Geometry check sheet. Reference: the model listing, model coordinates, mm. A direction names the side the tool comes from. Give positions to 0.01 mm unless a question says otherwise; leave off trailing zeros. Loops run counter-clockwise (first coordinate to the right, second up) from the corner with the lowest first, then second, coordinate; pieces in that order, holes last. Notation, with made-up numbers: (70.25, -39.75) -> (97.25, -39.75) arc R21 ccw to (97.25, -3.75) -> close; hole circle Ø3 at (50, 46.25). An arc over 180 degrees is marked (long way). Answer as a JSON object with one key per item and string values.
from build123d import *

# Parameters (mm, degrees)
BOSS_EXTRUDE1_DEPTH   = 3.175
F_6_CLEARANCE_HOLE1_D = 4.3053


with BuildPart() as part:
    # Sketch1 → Boss-Extrude1 (new body)
    with BuildSketch(Plane.XY):
        Polygon((866.156250481, 6490.011012461), (829.199261489, 6490.03953741), (829.199261489, 6625.537287847), (866.263292559, 6628.694971151), align=None)
        with BuildLine():
            Line((856.233206108, 6589.718701179), (856.176475752, 6516.218723072))
            ThreePointArc((856.176475752, 6516.218723072), (849.821576449, 6509.873626158), (843.476479535, 6516.22852546))
            Line((843.476479535, 6516.22852546), (843.533209891, 6589.728503567))
            ThreePointArc((843.533209891, 6589.728503567), (849.888109194, 6596.073600482), (856.233206108, 6589.718701179))
        make_face(mode=Mode.SUBTRACT)
    extrude(amount=BOSS_EXTRUDE1_DEPTH)

    # #6 Clearance Hole1 (through all)
    with Locations(Plane.XY.offset(3.175)):
        with Locations((859.90595224, 6619.187287847), (835.549261489, 6494.797137633)):
            Hole(F_6_CLEARANCE_HOLE1_D / 2)


solid = part.part
1) Draft check along X on faces 1 (the face through (840, 6560, 0)), 2 (the face through (829.199, 6557, 2)), 3 (the face through (835.83, 6496.93, 1.57)), 4 (the face through (858.91, 6617.28, 1.57)). Enter one of: pulls with the +X half, pulls with the -X half, needs draft (parallel to the pull), parting line crosses it, or undercut.
Geometry check:
{"face 1": "needs draft", "face 2": "pulls with the -X half", "face 3": "undercut", "face 4": "undercut"}
2) Tool access check on faces 5 (the face through (840, 6560, 3.175)), 6 (the face through (849.748, 6596.072, 1.565)). Record the directions out of +Z, -Z, +X, -X, +Y, -Y that give a thin tool (end or side, any length) a straight path to the whole face; none if there is none.
Geometry check:
{"face 5": "+Z, +X, -X, +Y, -Y", "face 6": "+Z, -Z"}
3) Section check A-A on y = 6533.5. Record the cut outline in (x, z) (3 decimals), plus the area to 3 significant figures.
Geometry check:
{"outline": "(829.199, 0) -> (843.49, 0) -> (843.49, 3.175) -> (829.199, 3.175) -> close; (856.19, 0) -> (866.19, 0) -> (866.19, 3.175) -> (856.19, 3.175) -> close", "area": "77.1 mm2"}
4) Section check B-B on x = 836. Record the cut outline in (y, z) (3 decimals), plus the area to 3 significant figures.
Geometry check:
{"outline": "(6490.034, 0) -> (6492.692, 0) -> (6492.692, 3.175) -> (6490.034, 3.175) -> close; (6496.902, 0) -> (6626.117, 0) -> (6626.117, 3.175) -> (6496.902, 3.175) -> close", "area": "419 mm2"}
5) Material ranges on line 1 along X through (y, z) = (6528, 1.3); line 2 along Y through (x, z) = (859, 0.3); line 3 along Y through (x, z) = (837.5, 2.3), recorded low to high. Write a range as from..to.
Geometry check:
{"line 1": "x = 829.2..843.49, 856.19..866.19", "line 2": "y = 6490.02..6617.23, 6621.14..6628.08", "line 3": "y = 6490.03..6493.89, 6495.71..6626.24"}
6) Section check D-D on x = 842. Record the cut outline in (y, z) (3 decimals).
Geometry check:
{"outline": "(6490.03, 0) -> (6626.628, 0) -> (6626.628, 3.175) -> (6490.03, 3.175) -> close"}
7) Section check C-C on z = 1.7. Record the cut outline in (x, y), plus the area to 3 significant figures.
Geometry check:
{"outline": "(829.2, 6490.04) -> (866.16, 6490.01) -> (866.26, 6628.69) -> (829.2, 6625.54) -> close; hole circle Ø4.31 at (835.55, 6494.8); hole (843.48, 6516.23) arc R6.35 ccw to (856.18, 6516.22) -> (856.23, 6589.72) arc R6.35 ccw to (843.53, 6589.73) -> close; hole circle Ø4.31 at (859.91, 6619.19)", "area": "3,980 mm2"}
